For this review, use the dimensioned drawing (mm, ordinates from the lowest corner) and the shaded views. Coordinates: 2 decimals unless noted, no trailing zeros. Write each loop counter-clockwise with the first axis right and the second up, starting at its lowest first coordinate (ties: lowest second). Pieces come first, ordered by that corner, then holes. Notation, with made-up numbers: (87.25, 28) -> (118.25, 28) arc R20 cw to (118.25, 63) -> close; hole circle Ø9 at (36.5, 42). An arc over 180 degrees is marked (long way). Put each result on its own line as item: value. Start each with the question number.
Item 1: Consider section A-A on y = 91.9. Give the boundary of the cut face in (x, z), and give its area (3 significant figures).
Item 2: Insertion check: P1, Ø8, axis at x = 128, z = 125, coming from the +Y side; P2, Ø3, axis at x = 96, y = 103, coming from the -Z side; P3, Ø4, axis at x = 27, y = 36, coming from the +Z side. Each pin has a flat end and moves straight along its axis. Give the tip position at first contact, or say it passes through.
Item 3: To check wall thickness, follow L1, parallel to Z at x = 17.5, y = 91; L2, parallel to Z at x = 91.5, y = 91.9; L3, parallel to Y at x = 90, z = 91. State the ranges of each line that lie inside material, in increasing order.
Item 4: The part is to be moulded in two halves that separate along Z. For the marked faces 1 and 2, say which applies: +Z half, -Z half, draft (parallel to the pull), parting line (faces both ways), or undercut.
Item 5: Consider section C-C on x = 138.5. Give the boundary of the cut face in (y, z), and give its area (3 significant figures).
Item 6: Consider section B-B on z = 134.5. Give the boundary of the cut face in (x, y).
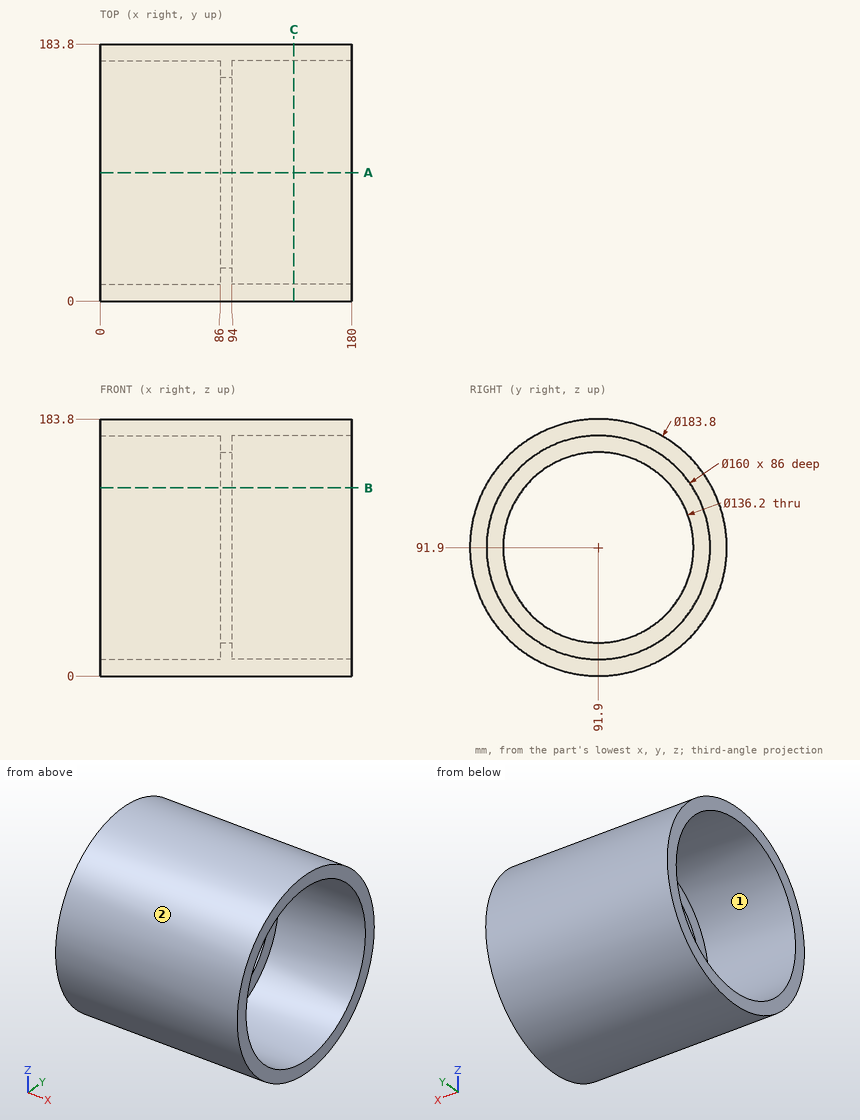
Return value:
1. outline: (0, 0) -> (180, 0) -> (180, 11.9) -> (94, 11.9) -> (94, 23.8) -> (86, 23.8) -> (86, 11.9) -> (0, 11.9) -> close; (0, 171.9) -> (86, 171.9) -> (86, 160) -> (94, 160) -> (94, 171.9) -> (180, 171.9) -> (180, 183.8) -> (0, 183.8) -> close
1. area: 4,470 mm^2
2. P1: y = 179.07
2. P2: z = 0.5
2. P3: z = 166.33
3. L1: 0 to 11.91, 171.89 to 183.8
3. L2: 0 to 23.8, 160 to 183.8
3. L3: 0 to 23.81, 159.99 to 183.8
4. face 1: undercut
4. face 2: parting line
5. outline: circle Ø183.8 at (91.9, 91.9); hole circle Ø160 at (91.9, 91.9)
5. area: 6,430 mm^2
6. outline: (0, 10.47) -> (180, 10.47) -> (180, 24.19) -> (94, 24.19) -> (94, 38.77) -> (86, 38.77) -> (86, 24.19) -> (0, 24.19) -> close; (0, 159.61) -> (86, 159.61) -> (86, 145.03) -> (94, 145.03) -> (94, 159.61) -> (180, 159.61) -> (180, 173.33) -> (0, 173.33) -> close
